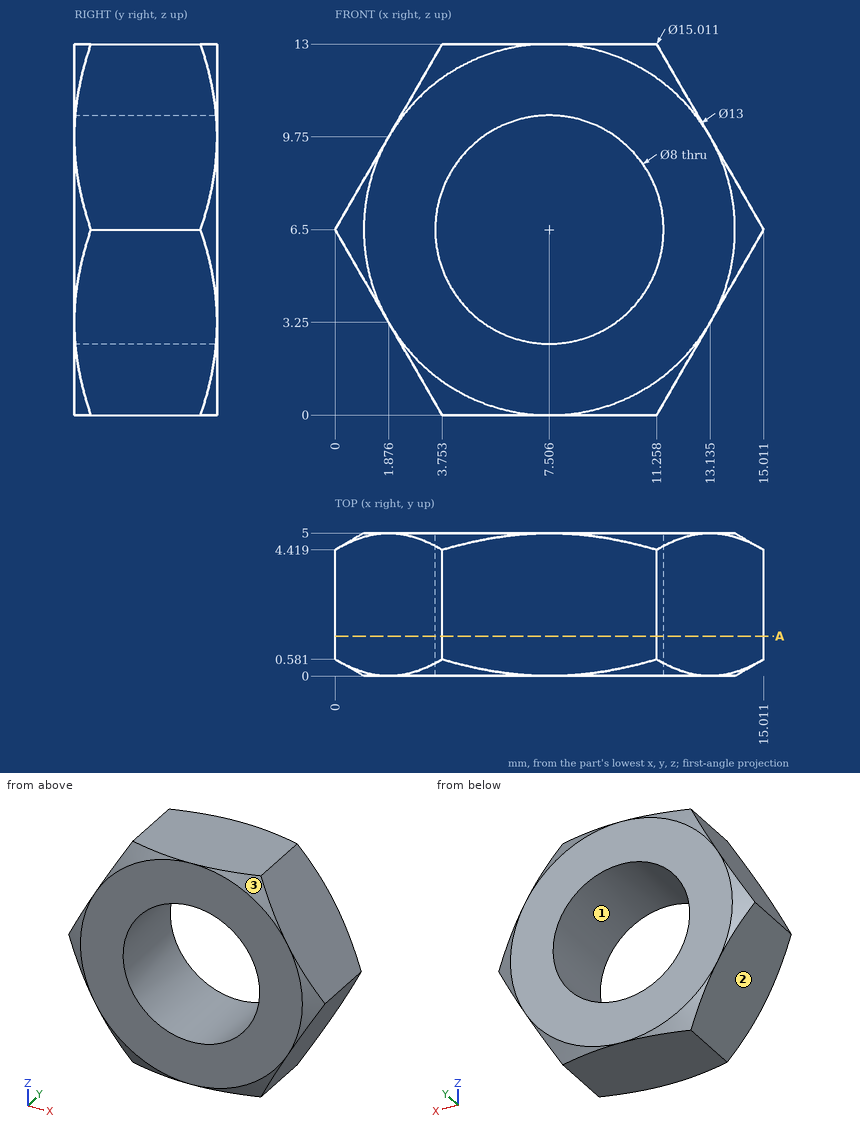
Input: dimensioned drawing with shaded views. Units: mm. Origin: part minimum x, y, z. Give positions to 0.01 mm unless a question says otherwise; leave off trailing zeros. Loops run counter-clockwise (first coordinate to the right, second up) from the corner with the lowest first, then second, coordinate; pieces in that order, holes last. Notation, with made-up numbers: (37, -38) -> (57, -38) arc R18 ccw to (57, -20) -> close; hole circle Ø7 at (-31, 74). An arc over 180 degrees is marked (long way). Return JSON: item names as keys, results as strings.
Item 1: Pin query (flat end, axial travel): P1, Ø1, axis at x = 2.5, y = 4.5, coming from the +Z side (1 decimal); P2, Ø2, axis at y = 2, z = 8, coming from the +X side. Return the tip coordinate at first contact, or that it passes through.
Filled in:
{"P1": "z = 11.7", "P2": "x = 14.72"}
Item 2: Mould query, pull axis Z, two halves, no side actions, for the marked faces 1, 2 and 3. Classes: released by +Z, released by -Z, zero draft, split by the parting line, or undercut.
Filled in:
{"face 1": "undercut", "face 2": "released by -Z", "face 3": "released by +Z"}
Item 3: Section A-A, the plane y = 1.4. Output: boundary loops of the cut face in (x, z) (1 decimal).
Filled in:
{"outline": "(0, 6.5) -> (3.8, 0) -> (11.3, 0) -> (15, 6.5) -> (11.3, 13) -> (3.8, 13) -> close; hole circle Ø8 at (7.5, 6.5)"}
Item 4: Line query: line 1 (Z direction, x = 6.5, y = 1.75); line 2 (X direction, y = 3.6, z = 7) (1 decimal); line 3 (X direction, y = 3.1, z = 5.25) (1 decimal). Output: solid intervals per line, ascending.
Filled in:
{"line 1": "0 to 2.63, 10.37 to 13", "line 2": "0.3 to 3.5, 11.5 to 14.7", "line 3": "0.7 to 3.7, 11.3 to 14.3"}
